Work out the finished part from the listing and answer in its coordinate system (mm). Face numbers are marked on the shaded views. Coordinates: 2 decimals unless noted, no trailing zeros. Order: outer loops, then holes, each group sorted by start corner. A loop starts at its lowest first (then second) coordinate and runs counter-clockwise, first axis right, second up. Notation, with made-up numbers: (38, -15) - (71, -15) arc R9 cw to (71, -5) - close; hole circle Ø9 at (4, -6.75). An arc over 180 degrees is marked (long way). Answer as a JSON object with one key per item and string values. Group by question number.
1) Section B-B (x = 46.5) is taken. Give the vertices of the cut face in (y, z), plus the area to 3 significant figures.
2) Section C-C (z = 1.45) is taken. Count the separate pieces of the cut face and the enclosed holes in it, plus the area to 3 significant figures.
3) Section A-A (x = 22) is taken. Give the vertices of the cut face in (y, z).
4) The mould has two halves that part along Y. Classify the marked faces 1, 2 and 3: released by +Y, released by -Y, zero draft, split by the parting line, or undercut.
5) Each of these flat-tipped pins is pushed along its axis until it touches: P1, Ø1, axis at y = 1.5, z = 2.5, coming from the -X side; P2, Ø12.5, axis at x = 100, y = 0, coming from the -Z side. Where does it stop, or does it pass through?
6) Find the intervals of material crossed by line 1 along Y through (x, z) = (100, 3.7); line 2 along Y through (x, z) = (0, 3.55); line 3 along X through (y, z) = (2.5, 0.3), in increasing order.
from build123d import *

# Parameters (mm, degrees)
EXTRUDE_1_DEPTH     = 5
SKETCH_2_R          = 3.15
CUT_EXTRUDE_1_DEPTH = 112.655720857
SKETCH_3_R          = 7.7
CUT_EXTRUDE_2_DEPTH = 112.655720857
CUT_EXTRUDE_3_DEPTH = 112.655720857
EXTRUDE_1_2_DEPTH   = 5
FILLET_1_R          = 1.6


with BuildPart() as part:
    # 草图1 → Extrude 1 (new body)
    with BuildSketch(Plane.XY):
        with BuildLine():
            Line((-0.18, -8.99819982), (99.78, -10.99779978))
            ThreePointArc((99.78, -10.99779978), (111, 0), (99.78, 10.99779978))
            Line((99.78, 10.99779978), (-0.18, 8.99819982))
            ThreePointArc((-0.18, 8.99819982), (-9, 0), (-0.18, -8.99819982))
        make_face()
    extrude(amount=EXTRUDE_1_DEPTH)

    # 草图2 → 切除-拉伸1 (cut, through all)
    with BuildSketch(Plane.XY.offset(5)):
        Circle(SKETCH_2_R)
    extrude(amount=-CUT_EXTRUDE_1_DEPTH, mode=Mode.SUBTRACT)

    # 草图3 → 切除-拉伸2 (cut, through all)
    with BuildSketch(Plane.XY.offset(5)):
        with Locations((100, 0)):
            Circle(SKETCH_3_R)
    extrude(amount=-CUT_EXTRUDE_2_DEPTH, mode=Mode.SUBTRACT)

    # 草图4 → 切除-拉伸3 (cut, through all)
    with BuildSketch(Plane.XY.offset(5)):
        with BuildLine():
            Line((7.381817961, 5.148666195), (86.596154404, 6.733269877))
            ThreePointArc((86.596154404, 6.733269877), (85, 0), (86.596154404, -6.733269877))
            Line((86.596154404, -6.733269877), (7.381817961, -5.148666195))
            ThreePointArc((7.381817961, -5.148666195), (9, 0), (7.381817961, 5.148666195))
        make_face()
    extrude(amount=-CUT_EXTRUDE_3_DEPTH, mode=Mode.SUBTRACT)

    # 草图5 → Extrude 1 2 (add, through all)
    with BuildSketch(Plane.XY.offset(5)):
        Polygon((6.589719105, 3.31220781), (32.616219561, -7.91350871), (50.030218058, 3.564346875), (66.717027477, -8.776023625), (87.697436335, 5.063785493), (85.494872472, 8.40275426), (66.847877099, -3.897809486), (50.161963875, 8.441898252), (32.217750586, -3.385430707), (8.173916817, 6.985124581), align=None)
    extrude(amount=-EXTRUDE_1_2_DEPTH)

    # 圆角1
    fillet_1_edges = [part.edges().sort_by_distance(p)[0] for p in [
        (7.381817961, -5.148666195, 2.5),
        (86.596154404, -6.733269877, 2.5),
        (27.121513236, -5.543539083, 2.5),
        (35.944131409, -5.720026748, 2.5),
        (63.325320924, -6.267760096, 2.5),
        (70.307680542, -6.407435226, 2.5),
        (82.850434699, 6.658340495, 2.5),
        (53.37111962, 6.068636241, 2.5),
        (46.348147736, 5.928148703, 2.5),
        (12.20786682, 5.245206483, 2.5),
        (32.217750586, -3.385430707, 2.5),
        (66.847877099, -3.897809486, 2.5),
        (85.430653574, 3.56849334, 2.5),
        (50.030218058, 3.564346875, 2.5),
        (8.669944071, 2.414967867, 2.5),
    ]]
    fillet(fillet_1_edges, radius=FILLET_1_R)


solid = part.part
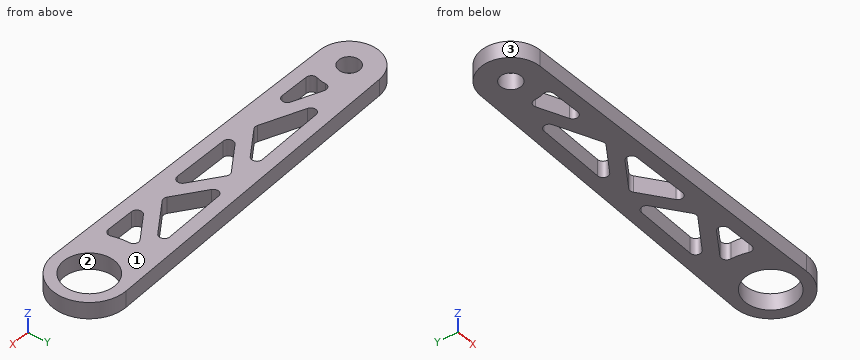
Report:
{
 "1": {"outline": "(-9.93, 0) - (-5.93, 0) - (-5.93, 5) - (-9.93, 5) - close; (1.24, 0) - (9.93, 0) - (9.93, 5) - (1.24, 5) - close", "area": "63.5 mm²"},
 "2": {"separate pieces": "1", "enclosed holes": "7", "area": "1,570 mm²"},
 "3": {"outline": "(-9.44, 0) - (1.02, 0) - (1.02, 5) - (-9.44, 5) - close; (5.44, 0) - (9.44, 0) - (9.44, 5) - (5.44, 5) - close"},
 "4": {"face 1": "zero draft", "face 2": "undercut", "face 3": "split by the parting line"},
 "5": {"P1": "stops at x = -8.94", "P2": "passes through"},
 "6": {"line 1": "y = -11 to -7.7, 7.7 to 11", "line 2": "y = -9 to -3.15, 3.15 to 9", "line 3": "x = -8.65 to -1.92, 1.92 to 18.67, 41.15 to 48.42, 51.47 to 58.2, 76.55 to 92.72, 107.28 to 110.71"}
}
